Input: part model. Units: mm. Frame: model coordinates. A direction names the side the tool comes from. Round coordinates to 2 decimals unless told otherwise and drop trailing zeros. Order: outer loops, then holes, each group sorted by start corner. A loop starts at its lowest first (then second) coordinate and runs counter-clockwise, first axis right, second up. Notation, with made-up numbers: (34, 72.5) - (78, 72.5) arc R28 cw to (78, 108.5) - close; hole circle Ø11 at (-21.75, 28.25). An arc over 180 degrees is marked (long way). One line per item, written item: value. Start each with the question number.
Autodesk Inventor part; units mm, degrees
ref_plane "YZ Plane" through (0, 0, 0) normal (1, 0, 0) x (0, 1, 0)
ref_plane "XZ Plane" through (0, 0, 0) normal (0, 1, 0) x (-1, 0, 0)
ref_plane "XY Plane" through (0, 0, 0) normal (0, 0, 1) x (1, 0, 0)
sketch "スケッチ1" plane through (0, 0, 0) normal (1, 0, 0) x (0, 1, 0)
  line L0 (8.6678, 22.4898) -> (-7.9322, 22.4898)
  line L1 (-7.9322, 22.4898) -> (-7.9322, -15.0102)
  line L2 (-7.9322, -15.0102) -> (8.6678, -15.0102)
  line L3 (8.6678, -15.0102) -> (8.6678, 22.4898)
  line L4 (8.6678, 22.4898) -> (6.6678, 22.4898)
  line L5 (6.6678, 22.4898) -> (6.6678, -0.0102)
  line L6 (6.6678, -0.0102) -> (8.6678, -0.0102)
  line L7 (8.6678, -0.0102) -> (8.6678, 22.4898)
  line L8 (-7.9322, 22.4898) -> (-5.9322, 22.4898)
  line L9 (-5.9322, 22.4898) -> (-5.9322, -0.0102)
  line L10 (-5.9322, -0.0102) -> (-7.9322, -0.0102)
  line L11 (-7.9322, -0.0102) -> (-7.9322, 22.4898)
  line L12 (8.6678, 22.4898) -> (-7.9322, 22.4898)
  line L13 (-7.9322, 22.4898) -> (-7.9322, 24.4898)
  line L14 (-7.9322, 24.4898) -> (8.6678, 24.4898)
  line L15 (8.6678, 24.4898) -> (8.6678, 22.4898)
  circle A0 centre (5.6678, -10.0102) radius 1.5
  circle A1 centre (-4.9322, -10.0102) radius 1.5
  point P0 (0, 0)
  dimension "d1" = 2
  dimension "d2" = 2
  dimension "d3" = 15
  dimension "d4" = 22.5
  dimension "d5" = 2
  dimension "d6" = 3
  dimension "d7" = 3
  dimension "d8" = 5
  dimension "d9" = 5
  dimension "d10" = 3
  dimension "d11" = 3
  dimension "d25" = 12.6
  dimension "d26" = 16.6
extrude "押し出し1" add sketch "スケッチ1" against normal blind 4
extrude "押し出し2" add sketch "スケッチ1" along normal blind 5 contours L3 L6 L5 L0 | L0 L13 L14 L15 | L9 L10 L1 L0
sketch "スケッチ2" plane through (0, 0, 0) normal (1, 0, 0) x (0, 0, -1)
  circle A0 centre (-17.2898, 1.4678) radius 3.5
  line L0 (-24.4898, 8.6678) -> (-24.4898, -7.9322)
  line L1 (0.0102, 8.6678) -> (-24.4898, 8.6678)
  line L2 (-24.4898, -7.9322) -> (0.0102, -7.9322)
  point P0 (0, 0)
  dimension "d16" = 7
  dimension "d17" = 7.2
  dimension "d18" = 7.2
  dimension "d19" = 9.4
extrude "押し出し3" cut sketch "スケッチ2" against normal blind 5
sketch "スケッチ3" plane through (0, 0, 0) normal (1, 0, 0) x (0, 0, -1)
  line L0 (-24.4898, 8.6678) -> (15.0102, 8.6678)
  line L1 (0.0102, -7.9322) -> (15.0102, -7.9322)
  line L2 (0, 8.6678) -> (5, 8.6678)
  line L3 (5, 8.6678) -> (5, -7.9322)
  line L4 (5, -7.9322) -> (0, -7.9322)
  line L5 (0, -7.9322) -> (0, 8.6678)
  point P0 (0, 0)
  dimension "d22" = 5
extrude "押し出し4" add sketch "スケッチ3" along normal blind 5
properties part number "armpart2"
1. Section B-B (z = 18.5). Return the cut outline in (x, y), then the cut area to 3 significant figures.
2. Pin query (flat end, axial travel): pin 1 (4 mm diameter, centred on y = 2, z = 11.5, fed in from +X); pin 2 (2.5 mm diameter, centred on x = 2.5, y = 0, fed in from -Z); pin 3 (5 mm diameter, centred on y = -4.93, z = -10.01, fed in from -X). Return the tip coordinate at first contact, or that it passes through.
3. Set-up query: faces 1 (the face through (-4, 0, 5)), 2 (the face through (2, 0, 0)), 3 (the face through (2, 0, -5)). Return all of +Z, -Z, +X, -X, +Y, -Y with unobstructed straight access to the full face (end or side cutting, diameter ignored); none if empty.
4. Pull-direction query (Z, two-part tool) for faces 4 (the face through (0, -7.932, 5)), 5 (the face through (2, 0, 22.49)), 6 (the face through (1, 0, 24.49)); classes: released by +Z, released by -Z, zero draft, split by the parting line, or undercut.
5. Line query: line 1 (Z direction, x = 2.5, y = 3); line 2 (Z direction, x = -0.25, y = -5); line 3 (Y direction, x = -1.25, z = -11). Output: solid intervals per line, ascending. Write a range as from..to.
6. Section A-A (y = -5.25). Return the cut outline in (x, z).
7. Section D-D (z = 0.5). Return the cut outline in (x, y), then the cut area to 3 significant figures.
8. Section C-C (x = 1). Return the cut outline in (y, z).
Solved:
1. outline: (-4, -7.93) - (5, -7.93) - (5, -5.93) - (0, -5.93) - (0, -1.82) - (-4, -1.82) - close; (-4, 4.75) - (0, 4.75) - (0, 6.67) - (5, 6.67) - (5, 8.67) - (-4, 8.67) - close
1. area: 60.1 mm²
2. pin 1: stops at x = 0
2. pin 2: stops at z = -5
2. pin 3: stops at x = -4
3. face 1: +Z, -Z, -X, +Y, -Y
3. face 2: +X
3. face 3: -Z, +X, +Y, -Y
4. face 4: zero draft
4. face 5: undercut
4. face 6: released by +Z
5. line 1: z = -5..0, 22.49..24.49
5. line 2: z = -15.01..-11.51, -8.51..24.49
5. line 3: y = -7.93..-6.06, -3.81..4.54, 6.79..8.67
6. outline: (-4, -15.01) - (0, -15.01) - (0, -11.48) - (-4, -11.48) - close; (-4, -8.54) - (0, -8.54) - (0, -5) - (5, -5) - (5, 0) - (0, 0) - (0, 22.49) - (5, 22.49) - (5, 24.49) - (-4, 24.49) - close
7. outline: (-4, -7.93) - (5, -7.93) - (5, -5.93) - (0, -5.93) - (0, 6.67) - (5, 6.67) - (5, 8.67) - (-4, 8.67) - close
7. area: 86.4 mm²
8. outline: (-7.93, -5) - (8.67, -5) - (8.67, 24.49) - (-7.93, 24.49) - close; hole (-5.93, 0) - (6.67, 0) - (6.67, 22.49) - (-5.93, 22.49) - close
